```python
from build123d import *

# Parameters (mm, degrees)
SKETCH2_W           = 812.8
SKETCH2_H           = 812.8
BOSS_EXTRUDE1_DEPTH = 1219.2
SKETCH3_W           = 912.8
SKETCH3_H           = 912.8
SKETCH3_W_2         = 812.8
SKETCH3_H_2         = 812.8
BOSS_EXTRUDE2_DEPTH = 100
CHAMFER4_SIZE       = 880
CHAMFER4_SIZE2      = 373.537838264


with BuildPart() as part:
    # Sketch2 → Boss-Extrude1 (new body)
    with BuildSketch(Plane(origin=(0, 0, 0), x_dir=(1, 0, 0), z_dir=(0, 1, 0))):
        with Locations((406.4, 406.4)):
            Rectangle(SKETCH2_W, SKETCH2_H)
    extrude(amount=BOSS_EXTRUDE1_DEPTH)

    # Sketch3 → Boss-Extrude2 (add)
    with BuildSketch(Plane(origin=(0, 100, 0), x_dir=(1, 0, 0), z_dir=(0, 1, 0))):
        with Locations((406.4, 406.4)):
            Rectangle(SKETCH3_W, SKETCH3_H)
        with Locations((406.4, 406.4)):
            Rectangle(SKETCH3_W_2, SKETCH3_H_2, mode=Mode.SUBTRACT)
    extrude(amount=BOSS_EXTRUDE2_DEPTH)

    # Chamfer4
    chamfer4_edges = [part.edges().sort_by_distance(p)[0] for p in [
        (0, 1219.2, -406.4),
    ]]
    chamfer4_side = [part.faces().sort_by_distance(p)[0] for p in [
        (0, 709.6, -406.4),
    ]]
    chamfer(chamfer4_edges, length=CHAMFER4_SIZE, length2=CHAMFER4_SIZE2, reference=chamfer4_side[0])


solid = part.part
```
Model file for the job. Use its own axes, mm. A direction names the side the tool comes from. Coordinates: 2 decimals unless noted, no trailing zeros. Loops run counter-clockwise (first coordinate to the right, second up) from the corner with the lowest first, then second, coordinate; pieces in that order, holes last. Notation, with made-up numbers: (56.5, 55) - (76.5, 55) arc R27 cw to (76.5, 84) - close; hole circle Ø2 at (-38.75, 1). An arc over 180 degrees is marked (long way). Answer as a JSON object with one key per item and string values. Group by question number.
(1) Tool access for faces 1 (the face through (0, 269, -401)), 2 (the face through (401, 49, -812.8)), 3 (the face through (401, 49, 0)), 4 (the face through (812.8, 702, -401)), 5 (the face through (491, 702, 0)): list every direction of +Z, -Z, +X, -X, +Y, -Y with a clear straight run to the whole face (end or side of a thin tool).
(2) Cut at B-B (z = -540). Give the cut face in (x, y), then the cut area to 3 significant figures.
(3) Flat gauge pins, fed straight in: pin 1 (6 mm diameter, centred on y = 852.5, z = -472, fed in from -X); pin 2 (10 mm diameter, centred on x = 347.5, y = 551.5, fed in from -Z); pin 3 (2 mm diameter, centred on x = 219, y = 428, fed in from +Z). Where does each tip first touch, or does it go through?
(4) Cut at A-A (x = 426.5). Give the cut face in (y, z), then the cut area to 3 significant figures.
(5) Cut at C-C (y = 323). Give the cut face in (x, z), then the cut area to 3 significant figures.
(6) Probe line 1 along Z through (x, y) = (194.5, 573); line 2 along X through (y, z) = (780, -76.5); line 3 along X through (y, z) = (860, -493). List the from-to ranges inside material, lowest first.
(7) Cut at D-D (x = 106). Give the cut face in (y, z).
Geometry says:
{
 "1": {"face 1": "+Z, -Z, -X, +Y", "face 2": "-Z, +X, -X, -Y", "face 3": "+Z, +X, -X, -Y", "face 4": "+Z, -Z, +X, +Y", "face 5": "+Z, +X, -X, +Y"},
 "2": {"outline": "(-50, 100) - (0, 100) - (0, 0) - (812.8, 0) - (812.8, 100) - (862.8, 100) - (862.8, 200) - (812.8, 200) - (812.8, 1219.2) - (373.54, 1219.2) - (0, 339.2) - (0, 200) - (-50, 200) - close", "area": "837,000 mm^2"},
 "3": {"pin 1": "stops at x = 216.61", "pin 2": "stops at z = -812.8", "pin 3": "stops at z = 0"},
 "4": {"outline": "(0, -812.8) - (100, -812.8) - (100, -862.8) - (200, -862.8) - (200, -812.8) - (1219.2, -812.8) - (1219.2, 0) - (200, 0) - (200, 50) - (100, 50) - (100, 0) - (0, 0) - close", "area": "1,000,000 mm^2"},
 "5": {"outline": "(0, -812.8) - (812.8, -812.8) - (812.8, 0) - (0, 0) - close", "area": "661,000 mm^2"},
 "6": {"line 1": "z = -812.8 to 0", "line 2": "x = 187.11 to 812.8", "line 3": "x = 221.07 to 812.8"},
 "7": {"outline": "(0, -812.8) - (100, -812.8) - (100, -862.8) - (200, -862.8) - (200, -812.8) - (588.92, -812.8) - (588.92, 0) - (200, 0) - (200, 50) - (100, 50) - (100, 0) - (0, 0) - close"}
}
